Here's the drawing with two shaded views (mm, measured from the low corner). I have some questions. Give positions to 0.01 mm unless a question says otherwise; leave off trailing zeros. Order: outer loops, then holes, each group sorted by start corner. A loop starts at its lowest first (then second) coordinate and runs counter-clockwise, first axis right, second up. Notation, with made-up numbers: M 89.5,-19.5 L 145.5,-19.5 A16 cw 145.5,11.5 Z; hole C 58,-24 d10. An arc over 180 degrees is marked long. Use a Markdown table: item, result. Add a question column.
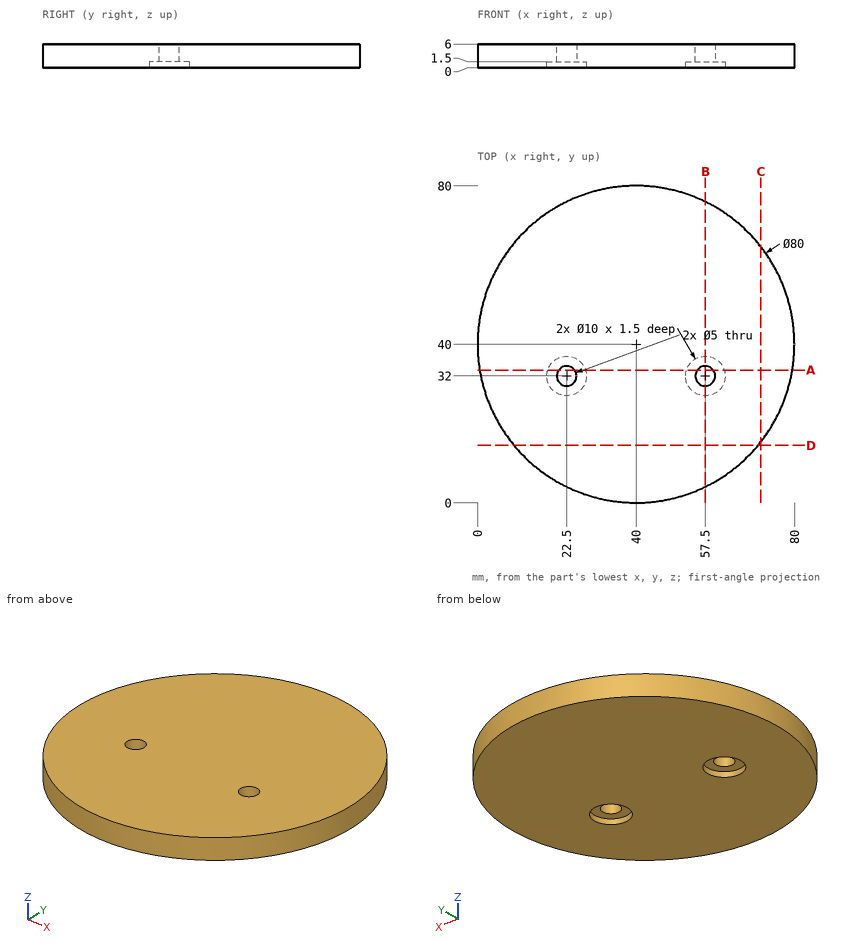
1) Suppose I cut it at A-A on y = 33.5. Please give me the cut outline in (x, z), and give its area (3 significant figures).
2) Suppose I cut it at B-B on x = 57.5. Please give me the cut outline in (y, z).
3) Please list where these lines run through material, in increasing order: line 1 (Y direction, x = 57.5, z = 4.05); line 2 (Y direction, x = 22.5, z = 0.5); line 3 (Y direction, x = 68, z = 1.8). Write a range as from..to.
4) For pin 1 (2 mm diameter, centred on x = 21, y = 28.5, fed in from -Z); pin 2 (3 mm diameter, centred on x = 69.5, z = 2, fed in from -Y); pin 3 (4.5 mm diameter, centred on x = 57.5, y = 32, fed in from +Z), each with a flat end and sliding along its axis, tell me the tip position at first contact or that it passes through.
5) Suppose I cut it at D-D on y = 14.5. Please give me the cut outline in (x, z), and give its area (3 significant figures).
6) Suppose I cut it at C-C on x = 71.5. Please give me the cut outline in (y, z), and give its area (3 significant figures).
Values found:
| question | item | result |
|---|---|---|
| 1 | outline | M 0.53,0 L 17.73,0 L 17.73,1.5 L 20.5,1.5 L 20.5,6 L 0.53,6 Z; M 24.5,1.5 L 27.27,1.5 L 27.27,0 L 52.73,0 L 52.73,1.5 L 55.5,1.5 L 55.5,6 L 24.5,6 Z; M 59.5,1.5 L 62.27,1.5 L 62.27,0 L 79.47,0 L 79.47,6 L 59.5,6 Z |
| 1 | area | 409 mm^2 |
| 2 | outline | M 4.03,0 L 27,0 L 27,1.5 L 29.5,1.5 L 29.5,6 L 4.03,6 Z; M 34.5,1.5 L 37,1.5 L 37,0 L 75.97,0 L 75.97,6 L 34.5,6 Z |
| 3 | line 1 | y = 4.03..29.5, 34.5..75.97 |
| 3 | line 2 | y = 4.03..27, 37..75.97 |
| 3 | line 3 | y = 11.43..68.57 |
| 4 | pin 1 | stops at z = 1.5 |
| 4 | pin 2 | stops at y = 11.43 |
| 4 | pin 3 | passes through |
| 5 | outline | M 9.18,0 L 70.82,0 L 70.82,6 L 9.18,6 Z |
| 5 | area | 370 mm^2 |
| 6 | outline | M 15.35,0 L 64.65,0 L 64.65,6 L 15.35,6 Z |
| 6 | area | 296 mm^2 |
